Part model, mm, in its own coordinate system. A direction names the side the tool comes from. Give positions to 0.01 mm unless a question says otherwise; leave off trailing zeros. Write each loop counter-clockwise with the first axis right and the second up, starting at its lowest first coordinate (ties: lowest second). Pieces come first, ordered by that corner, then holes. Notation, with made-up numbers: M 80,9 L 94,9 A24 cw 94,39 Z; hole C -35.75,9 d8. An arc over 180 degrees is marked long. Use CSV: the item, a comma, the result in double quotes. Start each with the question number.
1. Mould opens along Z. For faces 4 (the face through (0.57, -0.03, -6.75)), 5 (the face through (3.298, -9.298, -29.525)), 6 (the face through (-0.508, 7, 0)) say: pulls with the +Z half, pulls with the -Z half, needs draft (parallel to the pull), parting line crosses it, or undercut.
2. Band-saw the part on C-C, the plane z = 11. List the corners of the cut face in (x, y).
3. Band-saw the part on B-B, the plane y = 23. List the corners of the cut face in (x, z).
4. Drill centre lines: line 1 along Z through (x, y) = (2.95, 0); line 2 along Z through (x, y) = (1.4, 0); line 3 along Y through (x, z) = (3.4, 0). Where is each one in solid material? Low to high. Write a range as from..to.
5. 3-axis set-ups, long thin cutter, end or side, ignore diameter. For faces 1 (the face through (0.57, 5.75, 10.77)), 2 (the face through (2.6, -1.29, 0.17)), 3 (the face through (3.048, -20.5, -22.8)): which of +Z, -Z, +X, -X, +Y, -Y reach the whole face in a straight line?
6. Band-saw the part on D-D, the plane y = 9. List the corners of the cut face in (x, z), then the cut area to 3 significant figures.
7. Drop flat-ended pins along their axis: pin 1 Ø2.5 at (y, z) = (0, 0) entering from -X; pin 2 Ø1 at (x, z) = (0, 1) entering from -Y; pin 3 Ø1.5 at (x, z) = (3, -7) entering from -Y. Give the stop position or say it passes through.
8. Band-saw the part on A-A, the plane x = 0.7. List the corners of the cut face in (y, z), then the cut area to 3 significant figures.
Autodesk Inventor part; units mm, degrees
ref_plane "YZ Plane" through (0, 0, 0) normal (1, 0, 0) x (0, 1, 0)
ref_plane "XZ Plane" through (0, 0, 0) normal (0, 1, 0) x (-1, 0, 0)
ref_plane "XY Plane" through (0, 0, 0) normal (0, 0, 1) x (1, 0, 0)
sketch "Sketch1" plane through (0, 0, 0) normal (1, 0, 0) x (0, 1, 0)
  circle A0 centre (0, 0) radius 30.48
  dimension "d0" = 60.96
extrude "Extrusion1" add sketch "Sketch1" along normal blind 3.048
sketch "Sketch2" plane through (3.048, 0, 0) normal (1, 0, 0) x (0, 0, -1)
  circle A0 centre (0, 0) radius 30.9541
extrude "Extrusion2" add sketch "Sketch2" along normal blind 0.508
sketch "Sketch3" plane through (0, 0, 0) normal (-1, 0, 0) x (0, 0, 1)
  circle A0 centre (0, 0) radius 30.9541
extrude "Extrusion3" add sketch "Sketch3" along normal blind 0.508
sketch "Sketch4" plane through (3.556, 0, 0) normal (1, 0, 0) x (0, 0, -1)
  circle A0 centre (0, 0) radius 1.3
  dimension "d7" = 2.6
hole "Hole1" at (3.556, 0, 0) direction (-1, 0, 0) diameter 2.6 end through all
sketch "Sketch5" plane through (3.556, 0, 0) normal (1, 0, 0) x (0, 0, -1)
  circle A0 centre (0, 0) radius 1.3
  circle A1 centre (-16.2, 0) radius 0.5
  circle A2 centre (0, 16.2) radius 0.5
  circle A3 centre (16.2, 0) radius 0.5
  circle A4 centre (0, -16.2) radius 0.5
  dimension "d19" = 1
  dimension "d20" = 1
  dimension "d21" = 1
  dimension "d22" = 1
hole "Hole2" at (3.556, 16.2, 0) at (3.556, -16.2, 0) at (3.556, 0, -16.2) at (3.556, 0, 16.2) direction (-1, 0, 0) diameter 1 end through all
sketch "Sketch6" plane through (-0.508, 0, 0) normal (-1, 0, 0) x (0, 0, 1)
  arc A0 (1.5256, -7.6067) -> (-1.5256, -7.6067) centre (0, -8.5367) ccw
  line L0 (1.5256, -7.6067) -> (10.0877, -14.0155)
  arc A1 (10.0877, -14.0155) -> (14.0155, -10.0877) centre (11.7691, -11.7691) ccw
  line L1 (14.0155, -10.0877) -> (7.6067, -1.5256)
  arc A2 (7.6067, 1.5256) -> (7.6067, -1.5256) centre (8.5367, 0) ccw
  line L2 (7.6067, 1.5256) -> (14.0155, 10.0877)
  arc A3 (14.0155, 10.0877) -> (10.0877, 14.0155) centre (11.7691, 11.7691) ccw
  line L3 (10.0877, 14.0155) -> (1.5256, 7.6067)
  arc A4 (-1.5256, 7.6067) -> (1.5256, 7.6067) centre (0, 8.5367) ccw
  line L4 (-1.5256, 7.6067) -> (-10.0877, 14.0155)
  arc A5 (-10.0877, 14.0155) -> (-14.0155, 10.0877) centre (-11.7691, 11.7691) ccw
  line L5 (-14.0155, 10.0877) -> (-7.6067, 1.5256)
  arc A6 (-7.6067, -1.5256) -> (-7.6067, 1.5256) centre (-8.5367, 0) ccw
  line L6 (-7.6067, -1.5256) -> (-14.0155, -10.0877)
  arc A7 (-14.0155, -10.0877) -> (-10.0877, -14.0155) centre (-11.7691, -11.7691) ccw
  line L7 (-10.0877, -14.0155) -> (-1.5256, -7.6067)
  circle A8 centre (12.339, -12.339) radius 0.75
  circle A9 centre (9.8641, -9.8641) radius 0.75
  circle A10 centre (7.3893, -7.3893) radius 0.75
  circle A11 centre (4.9144, -4.9144) radius 0.75
  circle A12 centre (12.339, 12.339) radius 0.75
  circle A13 centre (9.8641, 9.8641) radius 0.75
  circle A14 centre (7.3893, 7.3893) radius 0.75
  circle A15 centre (4.9144, 4.9144) radius 0.75
  circle A16 centre (-12.339, 12.339) radius 0.75
  circle A17 centre (-9.8641, 9.8641) radius 0.75
  circle A18 centre (-7.3893, 7.3893) radius 0.75
  circle A19 centre (-4.9144, 4.9144) radius 0.75
  circle A20 centre (-12.339, -12.339) radius 0.75
  circle A21 centre (-9.8641, -9.8641) radius 0.75
  circle A22 centre (-7.3893, -7.3893) radius 0.75
  circle A23 centre (-4.9144, -4.9144) radius 0.75
  circle A24 centre (0, 0) radius 3.6
  point P0 (0, 0)
extrude "Extrusion4" cut sketch "Sketch6" against normal blind 2.1844 contours A0 L7 A7 L6 A6 L5 A5 L4 A4 L3 A3 L2 A2 L1 A1 L0 | A8 | A9 | A10 | A11 | A12 | A13 | A14 | A15 | A16 | A17 | A18 | A19 | A20 | A21 | A22 | A23 | A24
properties part number "Wheel"
Output:
1,face 4,"undercut"
1,face 5,"parting line crosses it"
1,face 6,"needs draft"
2,outline,"M -0.51,-28.93 L 0,-28.93 L 0,-28.43 L 3.05,-28.43 L 3.05,-28.93 L 3.56,-28.93 L 3.56,28.93 L 3.05,28.93 L 3.05,28.43 L 0,28.43 L 0,28.93 L -0.51,28.93 L -0.51,14.47 L 1.68,14.47 L 1.68,6.06 L -0.51,6.06 L -0.51,-6.06 L 1.68,-6.06 L 1.68,-14.47 L -0.51,-14.47 Z"
3,outline,"M -0.51,-20.72 L 0,-20.72 L 0,-20 L 3.05,-20 L 3.05,-20.72 L 3.56,-20.72 L 3.56,20.72 L 3.05,20.72 L 3.05,20 L 0,20 L 0,20.72 L -0.51,20.72 Z"
4,line 1,"z = -30.48..-16.7, -15.7..-1.3, 1.3..15.7, 16.7..30.48"
4,line 2,"z = -30.48..-16.7, -15.7..-6.75, 6.75..15.7, 16.7..30.48"
4,line 3,"y = -30.95..-16.7, -15.7..-1.3, 1.3..15.7, 16.7..30.95"
5,face 1,"-X"
5,face 2,"+X, -X"
5,face 3,"none"
6,outline,"M -0.51,-29.62 L 0,-29.62 L 0,-29.12 L 3.05,-29.12 L 3.05,-29.62 L 3.56,-29.62 L 3.56,29.62 L 3.05,29.62 L 3.05,29.12 L 0,29.12 L 0,29.62 L -0.51,29.62 L -0.51,13.2 L 1.68,13.2 L 1.68,3.39 L -0.51,3.39 L -0.51,-3.39 L 1.68,-3.39 L 1.68,-13.2 L -0.51,-13.2 Z"
6,area,"195 mm²"
7,pin 1,"passes through"
7,pin 2,"stops at y = -30.95"
7,pin 3,"stops at y = -30.32"
8,outline,"C 0,0 d60.96; hole C -16.2,0 d1; hole M -14.02,-10.09 A2.81 ccw -10.09,-14.02 L -1.53,-7.61 A1.79 cw 1.53,-7.61 L 10.09,-14.02 A2.81 ccw 14.02,-10.09 L 7.61,-1.53 A1.79 cw 7.61,1.53 L 14.02,10.09 A2.81 ccw 10.09,14.02 L 1.53,7.61 A1.79 cw -1.53,7.61 L -10.09,14.02 A2.81 ccw -14.02,10.09 L -7.61,1.53 A1.79 cw -7.61,-1.53 Z; hole C 0,-16.2 d1; hole C 0,16.2 d1; hole C 16.2,0 d1"
8,area,"2,430 mm²"
